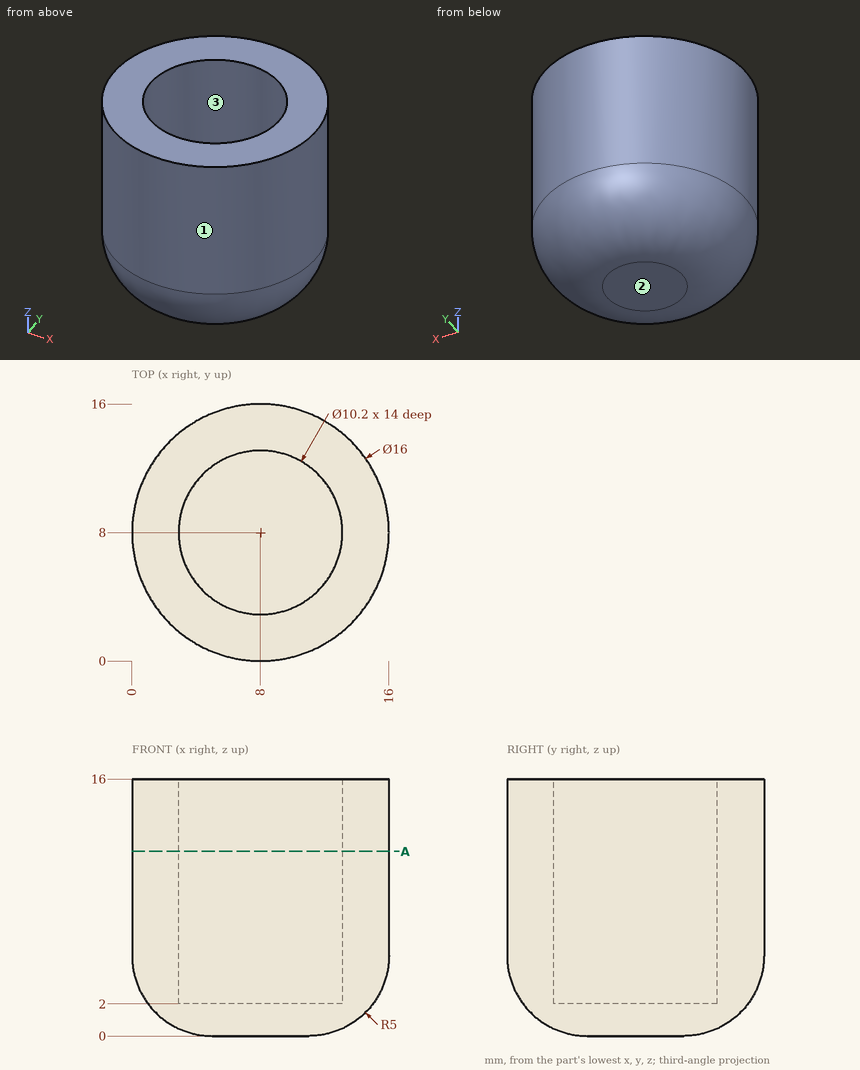
Check sheet for the drawn part. Datum: minimum x, y, z corner. Units: mm. Give positions to 0.01 mm unless a question says otherwise; leave off trailing zeros. Write each loop counter-clockwise with the first axis right and the second up, starting at its lowest first coordinate (ties: lowest second). Pieces come first, ordered by that corner, then holes. Notation, with made-up numbers: M 57,4 L 105,4 A18 ccw 105,35 Z; hole C -10.75,-5.5 d3. An arc over 180 degrees is marked long. One line per question, with ' | ' between items.
1. Mould release check, pull along Y, two halves, no side actions. Record for the marked faces 1, 2 and 3: released by +Y, released by -Y, zero draft, split by the parting line, or undercut.
Ans:
face 1: split by the parting line | face 2: zero draft | face 3: undercut
2. Scan lines: line 1 along Y through (x, z) = (8, 12.25); line 2 along Z through (x, y) = (7.5, 5.5); line 3 along Y through (x, z) = (6, 3). Record each from-to range of solid material in increasing order. Write a range as from..to.
Ans:
line 1: 0..2.9, 13.1..16 | line 2: 0..2 | line 3: 0.69..3.31, 12.69..15.31
3. Cross-section at A-A (z = 11.5). Enter the section's corners in (x, y).
Ans:
outline: C 8,8 d16; hole C 8,8 d10.2
4. Gauge pin test, flat ends, axial feed: pin 1 (1 mm diameter, centred on y = 4, z = 7.5, fed in from +X); pin 2 (3 mm diameter, centred on x = 10, y = 14, fed in from -Z); pin 3 (1 mm diameter, centred on x = 4, z = 7, fed in from +Y). Record the tip position at first contact, or that the pin passes through.
Ans:
pin 1: x = 15.19 | pin 2: z = 0.34 | pin 3: y = 15.19
